For this review, take the finished solid that the model builds, in its own axes (mm). A direction names the side the tool comes from. Round coordinates to 2 decimals unless told otherwise and drop trailing zeros. Loops run counter-clockwise (first coordinate to the right, second up) from the corner with the lowest first, then second, coordinate; pieces in that order, holes last. Notation, with made-up numbers: (76.5, -38.75) -> (131.5, -38.75) arc R33 ccw to (131.5, -10.75) -> close; hole circle Ø6 at (-35.5, -11.5). An arc over 180 degrees is marked (long way). Use one line per item in the form item = value. Start each with the question number.
from build123d import *

# Parameters (mm, degrees)
SKETCH1_R           = 35
BOSS_EXTRUDE1_DEPTH = 25
FILLET1_R           = 12.5
SKETCH2_R           = 11
CUT_EXTRUDE1_DEPTH  = 6.5
CUT_EXTRUDE2_START  = -6.5
SKETCH3_R           = 11
CUT_EXTRUDE2_DEPTH  = 6.5
SKETCH4_R           = 9
CUT_EXTRUDE3_DEPTH  = 53.841744861


with BuildPart() as part:
    # Sketch1 → Boss-Extrude1 (new body)
    with BuildSketch(Plane(origin=(0, 0, 0), x_dir=(1, 0, 0), z_dir=(0, 1, 0))):
        with Locations(Location((0, 0, 0), (0, 0, 270))):
            Circle(SKETCH1_R)
    extrude(amount=BOSS_EXTRUDE1_DEPTH)

    # Fillet1
    fillet1_edges = [part.edges().sort_by_distance(p)[0] for p in [
        (0, 0, -35),
        (0, 25, -35),
    ]]
    fillet(fillet1_edges, radius=FILLET1_R - 0.0001)  # a hair under: the kernel refuses the full size

    # Sketch2 → Cut-Extrude1 (cut)
    with BuildSketch(Plane(origin=(0, 25, 0), x_dir=(1, 0, 0), z_dir=(0, 1, 0))):
        with Locations(Location((0, 0, 0), (0, 0, 270))):
            Circle(SKETCH2_R)
    extrude(amount=-CUT_EXTRUDE1_DEPTH, mode=Mode.SUBTRACT)

    # Sketch3 → Cut-Extrude2 (cut)
    with BuildSketch(Plane.XZ.offset(CUT_EXTRUDE2_START)):
        with Locations(Location((0, 0, 0), (0, 0, 90))):
            Circle(SKETCH3_R)
    extrude(amount=CUT_EXTRUDE2_DEPTH, mode=Mode.SUBTRACT)

    # Sketch4 → Cut-Extrude3 (cut, through all)
    with BuildSketch(Plane.XZ.offset(-6.5)):
        with Locations(Location((0, 0, 0), (0, 0, 270))):
            Circle(SKETCH4_R)
    extrude(amount=-CUT_EXTRUDE3_DEPTH, mode=Mode.SUBTRACT)


solid = part.part
Item 1: Machinability: for faces 1 (the cylindrical face through (-10.74, 21.8, -2.38)), 2 (the cylindrical face through (10.74, 3.3, -2.38)), 3 (the cylindrical face through (2.703, 12.416, -8.584)), which of the approach directions +Z, -Z, +X, -X, +Y, -Y give a long, thin tool a straight path to every point of the face, cutting with its end or side? Answer none if there is none.
Item 2: Wall thickness on line 1 (X direction, y = 23.5, z = 3); line 2 (Y direction, x = 9, z = -5); line 3 (X direction, y = 9.75, z = 0): over which ranges is each line inside the solid? List them lowest first.
Item 3: Take a section at C-C on y = 4.25. Give the boundary of the cut face in (x, z).
Item 4: For P1, Ø1, axis at x = -4.5, z = -9, coming from the +Y side; P2, Ø1, axis at x = 22.5, z = -24.5, coming from the +Y side; P3, Ø3, axis at y = 16, z = -27.5, coming from the +X side; P4, Ø11, axis at x = -1.5, z = 0, coming from the -Y side, all flat-tipped, find the tip position at first contact; note any pin that passes through.
Item 5: Draft analysis for pull direction Z (two halves, no side actions). For faces 4 (the flat face through (9, 6.5, 2)), 5 (the flat face through (-10, 0, -5)), state which applies: +Z half, -Z half, draft (parallel to the pull), parting line (faces both ways), or undercut.
Results:
q1.face_1 = +Y
q1.face_2 = -Y
q1.face_3 = +Y, -Y
q2.line_1 = -28.28 to -10.58, 10.58 to 28.28
q2.line_2 = 6.5 to 18.5
q2.line_3 = -34.69 to -9, 9 to 34.69
q3.outline = circle Ø63.78 at (0, 0); hole circle Ø22 at (0, 0)
q4.P1 = 18.5
q4.P2 = 19.63
q4.P3 = 22.78
q4.P4 = through
q5.face_4 = undercut
q5.face_5 = draft
